```python
from build123d import *

# Parameters (mm, degrees)
SKETCH1_W           = 53.8988
SKETCH1_H           = 96.52
BOSS_EXTRUDE1_DEPTH = 31.6738
SKETCH2_R           = 6.35
BOSS_EXTRUDE2_DEPTH = 12.7
SKETCH3_R           = 3.4925
BOSS_EXTRUDE3_DEPTH = 110.49


with BuildPart() as part:
    # Sketch1 → Boss-Extrude1 (new body)
    with BuildSketch(Plane.XY):
        Rectangle(SKETCH1_W, SKETCH1_H)
    extrude(amount=BOSS_EXTRUDE1_DEPTH)

    # Sketch2 → Boss-Extrude2 (add)
    with BuildSketch(Plane(origin=(0, 48.26, 0), x_dir=(1, 0, 0), z_dir=(0, 1, 0))):
        with Locations(Location((14.2494, -12.7, 0), (0, 0, 90))):
            Circle(SKETCH2_R)
    extrude(amount=BOSS_EXTRUDE2_DEPTH)

    # Sketch3 → Boss-Extrude3 (add)
    with BuildSketch(Plane(origin=(0, 60.96, 0), x_dir=(1, 0, 0), z_dir=(0, 1, 0))):
        with Locations(Location((14.2494, -12.7, 0), (0, 0, 270))):
            Circle(SKETCH3_R)
    extrude(amount=BOSS_EXTRUDE3_DEPTH)


solid = part.part
```
Source: CAD feature listing. Evaluate the final solid. Frame: model axes, mm. A direction names the side the tool comes from. Round coordinates to 2 decimals unless told otherwise and drop trailing zeros. Loops run counter-clockwise (first coordinate to the right, second up) from the corner with the lowest first, then second, coordinate; pieces in that order, holes last. Notation, with made-up numbers: M 47,-28 L 79,-28 A19 ccw 79,5 Z; hole C 88,-34.75 d4. An arc over 180 degrees is marked long. Use a Markdown table: item, result. Add a question column.
1. Set-up query: faces 1 (the cylindrical face through (14.4, 115.43, 9.21)), 2 (the flat face through (0, -48.26, 16)). Return all of +Z, -Z, +X, -X, +Y, -Y with unobstructed straight access to the full face (end or side cutting, diameter ignored); none if empty.
2. Cut plane C-C, the plane y = 74.5. Output: boundary loops of the cut face in (x, z) (1 decimal).
3. Cut plane D-D, the plane z = 21.5. Output: boundary loops of the cut face in (x, y).
4. Cut plane A-A, the plane z = 12.7. Output: boundary loops of the cut face in (x, y), and give its area (3 significant figures).
5. Cut plane B-B, the plane x = -9. Output: boundary loops of the cut face in (y, z).
6. Contact query for flat-ended pins moving along their axis: pin 1 (3 mm diameter, centred on y = 50.5, z = 25.5, fed in from -X); pin 2 (5 mm diameter, centred on y = 147, z = 13, fed in from -X); pin 3 (1 mm diameter, centred on x = 15, y = 53, fed in from +Z). Output: stop coordinate, or through.
7. Ray query, line 1 along Y through (x, z) = (-11, 2); line 2 along X through (y, z) = (130.5, 13); line 3 along Z through (x, y) = (19, 53). Return the intervals inside material, ascending. Write a range as [from, to].
Solution:
| question | item | result |
|---|---|---|
| 1 | face 1 | +Y |
| 1 | face 2 | +Z, -Z, +X, -X, -Y |
| 2 | outline | C 14.2,12.7 d7 |
| 3 | outline | M -26.95,-48.26 L 26.95,-48.26 L 26.95,48.26 L -26.95,48.26 Z |
| 4 | outline | M -26.95,-48.26 L 26.95,-48.26 L 26.95,48.26 L 20.6,48.26 L 20.6,60.96 L 17.74,60.96 L 17.74,171.45 L 10.76,171.45 L 10.76,60.96 L 7.9,60.96 L 7.9,48.26 L -26.95,48.26 Z |
| 4 | area | 6,140 mm2 |
| 5 | outline | M -48.26,0 L 48.26,0 L 48.26,31.67 L -48.26,31.67 Z |
| 6 | pin 1 | passes through |
| 6 | pin 2 | stops at x = 10.76 |
| 6 | pin 3 | stops at z = 19.05 |
| 7 | line 1 | y = [-48.26, 48.26] |
| 7 | line 2 | x = [10.77, 17.73] |
| 7 | line 3 | z = [8.49, 16.91] |
